from build123d import *

# Parameters (mm, degrees)
SKETCH_1_R          = 80
EXTRUDE_1_DEPTH     = 4.5
CUT_EXTRUDE_1_REACH = 456.95
SKETCH_2_R          = 2


with BuildPart() as part:
    # 草图1 → 凸台-拉伸1 (new body)
    with BuildSketch(Plane.XY):
        Polygon((0, 0), (216.7, 0), (216.7, 176), (11.7, 400), (0, 400), align=None)
        with Locations((110, 110)):
            Circle(SKETCH_1_R, mode=Mode.SUBTRACT)
    extrude(amount=EXTRUDE_1_DEPTH)

    # 草图2 → 切除-拉伸1 (cut, up to next)
    with BuildSketch(Plane.XY.offset(4.5), mode=Mode.PRIVATE) as cut_extrude_1_sk1:
        with Locations((203.95, 20)):
            Circle(SKETCH_2_R)
    cut_extrude_1_tool1 = extrude(cut_extrude_1_sk1.sketch, amount=-CUT_EXTRUDE_1_REACH, mode=Mode.PRIVATE) & part.part
    # 草图2 → 切除-拉伸1 (cut, up to next)
    with BuildSketch(Plane.XY.offset(4.5), mode=Mode.PRIVATE) as cut_extrude_1_sk2:
        with Locations((203.95, 42)):
            Circle(SKETCH_2_R)
    cut_extrude_1_tool2 = extrude(cut_extrude_1_sk2.sketch, amount=-CUT_EXTRUDE_1_REACH, mode=Mode.PRIVATE) & part.part
    # 草图2 → 切除-拉伸1 (cut, up to next)
    with BuildSketch(Plane.XY.offset(4.5), mode=Mode.PRIVATE) as cut_extrude_1_sk3:
        with Locations((203.95, 130)):
            Circle(SKETCH_2_R)
    cut_extrude_1_tool3 = extrude(cut_extrude_1_sk3.sketch, amount=-CUT_EXTRUDE_1_REACH, mode=Mode.PRIVATE) & part.part
    # 草图2 → 切除-拉伸1 (cut, up to next)
    with BuildSketch(Plane.XY.offset(4.5), mode=Mode.PRIVATE) as cut_extrude_1_sk4:
        with Locations((203.95, 152)):
            Circle(SKETCH_2_R)
    cut_extrude_1_tool4 = extrude(cut_extrude_1_sk4.sketch, amount=-CUT_EXTRUDE_1_REACH, mode=Mode.PRIVATE) & part.part
    # 草图2 → 切除-拉伸1 (cut, up to next)
    with BuildSketch(Plane.XY.offset(4.5), mode=Mode.PRIVATE) as cut_extrude_1_sk5:
        with Locations((15, 30)):
            Circle(SKETCH_2_R)
    cut_extrude_1_tool5 = extrude(cut_extrude_1_sk5.sketch, amount=-CUT_EXTRUDE_1_REACH, mode=Mode.PRIVATE) & part.part
    # 草图2 → 切除-拉伸1 (cut, up to next)
    with BuildSketch(Plane.XY.offset(4.5), mode=Mode.PRIVATE) as cut_extrude_1_sk6:
        with Locations((15, 50)):
            Circle(SKETCH_2_R)
    cut_extrude_1_tool6 = extrude(cut_extrude_1_sk6.sketch, amount=-CUT_EXTRUDE_1_REACH, mode=Mode.PRIVATE) & part.part
    # 草图2 → 切除-拉伸1 (cut, up to next)
    with BuildSketch(Plane.XY.offset(4.5), mode=Mode.PRIVATE) as cut_extrude_1_sk7:
        with Locations((15, 300)):
            Circle(SKETCH_2_R)
    cut_extrude_1_tool7 = extrude(cut_extrude_1_sk7.sketch, amount=-CUT_EXTRUDE_1_REACH, mode=Mode.PRIVATE) & part.part
    # 草图2 → 切除-拉伸1 (cut, up to next)
    with BuildSketch(Plane.XY.offset(4.5), mode=Mode.PRIVATE) as cut_extrude_1_sk8:
        with Locations((15, 320)):
            Circle(SKETCH_2_R)
    cut_extrude_1_tool8 = extrude(cut_extrude_1_sk8.sketch, amount=-CUT_EXTRUDE_1_REACH, mode=Mode.PRIVATE) & part.part
    # 草图2 → 切除-拉伸1 (cut, up to next)
    with BuildSketch(Plane.XY.offset(4.5), mode=Mode.PRIVATE) as cut_extrude_1_sk9:
        with BuildLine():
            Line((57.106354887, 328.167238391), (68.171865568, 338.294156648))
            Line((68.171865568, 338.294156648), (81.674423243, 323.540142407))
            Line((81.674423243, 323.540142407), (70.608912563, 313.41322415))
            ThreePointArc((70.608912563, 313.41322415), (56.480626605, 314.038952433), (57.106354887, 328.167238391))
        make_face()
    cut_extrude_1_tool9 = extrude(cut_extrude_1_sk9.sketch, amount=-CUT_EXTRUDE_1_REACH, mode=Mode.PRIVATE) & part.part
    add(cut_extrude_1_tool1.solids().sort_by_distance((203.95, 20, 4.5))[0], mode=Mode.SUBTRACT)
    add(cut_extrude_1_tool2.solids().sort_by_distance((203.95, 42, 4.5))[0], mode=Mode.SUBTRACT)
    add(cut_extrude_1_tool3.solids().sort_by_distance((203.95, 130, 4.5))[0], mode=Mode.SUBTRACT)
    add(cut_extrude_1_tool4.solids().sort_by_distance((203.95, 152, 4.5))[0], mode=Mode.SUBTRACT)
    add(cut_extrude_1_tool5.solids().sort_by_distance((15, 30, 4.5))[0], mode=Mode.SUBTRACT)
    add(cut_extrude_1_tool6.solids().sort_by_distance((15, 50, 4.5))[0], mode=Mode.SUBTRACT)
    add(cut_extrude_1_tool7.solids().sort_by_distance((15, 300, 4.5))[0], mode=Mode.SUBTRACT)
    add(cut_extrude_1_tool8.solids().sort_by_distance((15, 320, 4.5))[0], mode=Mode.SUBTRACT)
    add(cut_extrude_1_tool9.solids().sort_by_distance((66.413044, 323.128888, 4.5))[0], mode=Mode.SUBTRACT)


solid = part.part
Can you work these out from the model? Positions are in its coordinate system, mm. A direction names the side the tool comes from. Give positions to 0.01 mm unless a question says otherwise; leave off trailing zeros. Loops run counter-clockwise (first coordinate to the right, second up) from the corner with the lowest first, then second, coordinate; pieces in that order, holes last. Notation, with made-up numbers: (71, 59) -> (90, 59) arc R8 cw to (90, 74) -> close; hole circle Ø1 at (16.5, 0). An arc over 180 degrees is marked (long way). Use one line per item in the form item = value.
1) If we section it at D-D (y = 215): Please give me the cut outline in (x, z), plus the area to 3 significant figures.
Answers:
outline = (0, 0) -> (181.01, 0) -> (181.01, 4.5) -> (0, 4.5) -> close
area = 815 mm²
2) For faces 1 (the face through (76.22, 318.55, 2.28)), 2 (the face through (56.63, 313.88, 2.28)), which set-ups out of +Z, -Z, +X, -X, +Y, -Y let a thin tool reach every point of the face, with its end or its side?
Answers:
face_1 = +Z, -Z, +Y
face_2 = +Z, -Z
3) If we section it at B-B (x = 110): Please give me the cut outline in (y, z).
Answers:
outline = (0, 0) -> (30, 0) -> (30, 4.5) -> (0, 4.5) -> close; (190, 0) -> (292.59, 0) -> (292.59, 4.5) -> (190, 4.5) -> close
4) I need wall thicknesses on line 1 along Y through (x, z) = (203.95, 3.3); line 2 along Y through (x, z) = (15, 2.65); line 3 along X through (y, z) = (151, 2.45). Which ranges of each line are inside material? Lowest first, please.
Answers:
line_1 = 0 to 18, 22 to 40, 44 to 128, 132 to 150, 154 to 189.93
line_2 = 0 to 28, 32 to 48, 52 to 298, 302 to 318, 322 to 396.39
line_3 = 0 to 41.31, 178.69 to 202.22, 205.68 to 216.7
5) If we section it at A-A (y = 110): Please give me the cut outline in (x, z).
Answers:
outline = (0, 0) -> (30, 0) -> (30, 4.5) -> (0, 4.5) -> close; (190, 0) -> (216.7, 0) -> (216.7, 4.5) -> (190, 4.5) -> close
6) Will this pin go through, and if not, where does the flat tip stop? pin 1 (1 mm diameter, centred on x = 40.5, z = 1.5, fed in from +Y).
Answers:
pin_1 = 369.08
7) If we section it at C-C (z = 3): Count the separate pieces of the cut face and the enclosed holes in it, plus the area to 3 significant figures.
Answers:
separate_pieces = 1
enclosed_holes = 9
area = 43,100 mm²
8) We'd pull the mould along Y, two halves only. Please class faces 3 (the face through (83, 203, 4.5)), 4 (the face through (150.13, 248.74, 2.22)), 5 (the face through (62.56, 333.16, 2.28)): released by +Y, released by -Y, zero draft, split by the parting line, or undercut.
Answers:
face_3 = zero draft
face_4 = released by +Y
face_5 = undercut
